Read the model definition and answer for the solid it produces. Units are mm, in the model's axes. A direction names the side the tool comes from. Coordinates: 2 decimals unless noted, no trailing zeros. Order: outer loops, then holes, each group sorted by start corner. A loop starts at its lowest first (then second) coordinate and runs counter-clockwise, first axis right, second up. Notation, with made-up numbers: (41, -11) - (82, -11) arc R25 ccw to (82, 3) - close; hole circle Ø7 at (42.5, 10.5). An arc over 180 degrees is marked (long way). Answer as a JSON object with one key per item and string values. Group by question number.
from build123d import *

# Parameters (mm, degrees)
F1_DEPTH = 67


# Not quite as in the source:
# - a feature names something its author has since deleted; it is built from what else it names


with BuildPart() as f1:
    # F0 (on Right) → F1 (new body)
    with BuildSketch(Plane.YZ):
        with BuildLine():
            Line((-23.8500006944, 31.9984000194), (-23.8500006944, -20.5015999806))
            Line((-23.8500006944, -20.5015999806), (30.1499993056, -20.5015999806))
            Line((30.1499993056, -20.5015999806), (30.1499993056, 0))
            Line((30.1499993056, 0), (21.0041528052, 0))
            ThreePointArc((21.0041528052, 0), (-15.527421475, 3.0121480227), (17.457689473, 19))
            Line((17.457689473, 19), (30.1499993056, 19))
            Line((30.1499993056, 19), (30.1499993056, 28.6984000194))
            Line((30.1499993056, 28.6984000194), (1.1499993056, 28.6984000194))
            Line((1.1499993056, 28.6984000194), (1.1499993056, 31.9984000194))
            Line((1.1499993056, 31.9984000194), (-23.8500006944, 31.9984000194))
        make_face()
    extrude(amount=F1_DEPTH)


solid = f1.part
1. Straight lines are drawn through the part: L1, parallel to Z at x = 9, y = 3.5; L2, parallel to Z at x = 51, y = 25.5; L3, parallel to Y at x = 8.5, z = 7. For each, find the intervals that lie inside material, in ascending order.
2. A cutting plane is placed at B-B on z = -2. Write down the section's boundary in (x, y), and give its area (3 significant figures).
3. Given pin 1 (23 mm diameter, centred on y = 3.15, z = 6.5, fed in from +X); pin 2 (14.5 mm diameter, centred on x = 47, y = 17, fed in from +Z); pin 3 (1.6 mm diameter, centred on x = 30, z = 31, fed in from +Y), each flat-ended and moving along its own axis, determine where each tip first touches the part or whether it passes through.
4. For a pull along Z with two mould halves and no side action, classify faces 4 (the flat face through (0, -15, 0)), 5 (the flat face through (33, 16, 28.698)), 6 (the flat face through (33, 24, 19)) as pulls with the +Z half, pulls with the -Z half, needs draft (parallel to the pull), parting line crosses it, or undercut.
5. A cutting plane is placed at A-A on y = 3.15. Write down the section's boundary in (x, z), and give its area (3 significant figures).
6. For faces 1 (the flat face through (33, 1.15, 30)), 2 (the flat face through (67, -15, 0)), 3 (the flat face through (33, 26, 0)), determine the directions among +Z, -Z, +X, -X, +Y, -Y from which every point of the face is accessible in a straight line to the end or side of a thin tool.
7. A cutting plane is placed at C-C on x = 15. Write down the section's boundary in (y, z), and give its area (3 significant figures).
8. A cutting plane is placed at D-D on z = 3.5. Write down the section's boundary in (x, y).
Derived:
{
 "1": {"L1": "z = -20.5 to -12.5, 25.5 to 28.7", "L2": "z = -20.5 to 0, 19 to 28.7", "L3": "y = -23.85 to -15.84"},
 "2": {"outline": "(0, -23.85) - (67, -23.85) - (67, -13.84) - (0, -13.84) - close; (0, 20.14) - (67, 20.14) - (67, 30.15) - (0, 30.15) - close", "area": "1,340 mm2"},
 "3": {"pin 1": "passes through", "pin 2": "stops at z = 28.7", "pin 3": "stops at y = 1.15"},
 "4": {"face 4": "needs draft", "face 5": "pulls with the +Z half", "face 6": "undercut"},
 "5": {"outline": "(0, -20.5) - (67, -20.5) - (67, -12.5) - (0, -12.5) - close; (0, 25.5) - (67, 25.5) - (67, 28.7) - (0, 28.7) - close", "area": "750 mm2"},
 "6": {"face 1": "+Z, +X, -X, +Y", "face 2": "+Z, -Z, +X, +Y, -Y", "face 3": "+X, -X, +Y"},
 "7": {"outline": "(-23.85, -20.5) - (30.15, -20.5) - (30.15, 0) - (21, 0) arc R19 cw (long way) to (17.46, 19) - (30.15, 19) - (30.15, 28.7) - (1.15, 28.7) - (1.15, 32) - (-23.85, 32) - close", "area": "1,430 mm2"},
 "8": {"outline": "(0, -23.85) - (67, -23.85) - (67, -15.61) - (0, -15.61) - close"}
}
